from build123d import *

# Parameters (mm, degrees)
SKETCH1_W           = 10.16
SKETCH1_H           = 5.08
SKETCH1_W_2         = 1
SKETCH1_H_2         = 1
BOSS_EXTRUDE2_DEPTH = 8
SKETCH2_W           = 10.16
SKETCH2_H           = 5.08
SKETCH2_R           = 0.5
BOSS_EXTRUDE3_DEPTH = 2
CHAMFER1_SIZE       = 0.2
CHAMFER2_SIZE       = 0.2


with BuildPart() as part:
    # Sketch1 → Boss-Extrude2 (new body)
    with BuildSketch(Plane.XY):
        Rectangle(SKETCH1_W, SKETCH1_H)
        with Locations((-1.27, 1.27)):
            Rectangle(SKETCH1_W_2, SKETCH1_H_2, mode=Mode.SUBTRACT)
        with Locations((-3.81, 1.27)):
            Rectangle(SKETCH1_W_2, SKETCH1_H_2, mode=Mode.SUBTRACT)
        with Locations((1.27, 1.27)):
            Rectangle(SKETCH1_W_2, SKETCH1_H_2, mode=Mode.SUBTRACT)
        with Locations((3.81, 1.27)):
            Rectangle(SKETCH1_W_2, SKETCH1_H_2, mode=Mode.SUBTRACT)
        with Locations((-1.27, -1.27)):
            Rectangle(SKETCH1_W_2, SKETCH1_H_2, mode=Mode.SUBTRACT)
        with Locations((1.27, -1.27)):
            Rectangle(SKETCH1_W_2, SKETCH1_H_2, mode=Mode.SUBTRACT)
        with Locations((3.81, -1.27)):
            Rectangle(SKETCH1_W_2, SKETCH1_H_2, mode=Mode.SUBTRACT)
        with Locations((-3.81, -1.27)):
            Rectangle(SKETCH1_W_2, SKETCH1_H_2, mode=Mode.SUBTRACT)
    extrude(amount=BOSS_EXTRUDE2_DEPTH)

    # Sketch2 → Boss-Extrude3 (add)
    with BuildSketch(Plane.XY.offset(8)):
        Rectangle(SKETCH2_W, SKETCH2_H)
        with Locations((-3.81, 1.27)):
            Circle(SKETCH2_R, mode=Mode.SUBTRACT)
        with Locations((-1.27, 1.27)):
            Circle(SKETCH2_R, mode=Mode.SUBTRACT)
        with Locations((1.27, 1.27)):
            Circle(SKETCH2_R, mode=Mode.SUBTRACT)
        with Locations((3.81, 1.27)):
            Circle(SKETCH2_R, mode=Mode.SUBTRACT)
        with Locations((-1.27, -1.27)):
            Circle(SKETCH2_R, mode=Mode.SUBTRACT)
        with Locations((1.27, -1.27)):
            Circle(SKETCH2_R, mode=Mode.SUBTRACT)
        with Locations((3.81, -1.27)):
            Circle(SKETCH2_R, mode=Mode.SUBTRACT)
        with Locations((-3.81, -1.27)):
            Circle(SKETCH2_R, mode=Mode.SUBTRACT)
    extrude(amount=BOSS_EXTRUDE3_DEPTH)

    # Chamfer1
    chamfer1_edges = [part.edges().sort_by_distance(p)[0] for p in [
        (-4.31, -1.27, 0),
        (-3.81, -1.77, 0),
        (-3.31, -1.27, 0),
        (-3.81, -0.77, 0),
        (-4.31, 1.27, 0),
        (-3.81, 0.77, 0),
        (-3.31, 1.27, 0),
        (-3.81, 1.77, 0),
        (-1.77, 1.27, 0),
        (-1.27, 0.77, 0),
        (-0.77, 1.27, 0),
        (-1.27, 1.77, 0),
        (0.77, 1.27, 0),
        (1.27, 0.77, 0),
        (1.77, 1.27, 0),
        (1.27, 1.77, 0),
        (0, 2.54, 0),
        (5.08, 0, 0),
        (0, -2.54, 0),
        (3.31, 1.27, 0),
        (3.81, 0.77, 0),
        (4.31, 1.27, 0),
        (3.81, 1.77, 0),
        (-5.08, 0, 0),
        (-1.77, -1.27, 0),
        (-1.27, -1.77, 0),
        (-0.77, -1.27, 0),
        (-1.27, -0.77, 0),
        (0.77, -1.27, 0),
        (1.27, -1.77, 0),
        (1.77, -1.27, 0),
        (1.27, -0.77, 0),
        (3.31, -1.27, 0),
        (3.81, -1.77, 0),
        (4.31, -1.27, 0),
        (3.81, -0.77, 0),
    ]]
    chamfer(chamfer1_edges, length=CHAMFER1_SIZE)

    # Chamfer2
    chamfer2_edges = [part.edges().sort_by_distance(p)[0] for p in [
        (-5.08, 0, 10),
        (0, -2.54, 10),
        (5.08, 0, 10),
        (0, 2.54, 10),
    ]]
    chamfer(chamfer2_edges, length=CHAMFER2_SIZE)


solid = part.part
Check sheet for the modelled part. Datum: model origin and axes. Units: mm. A direction names the side the tool comes from. Give positions to 0.01 mm unless a question says otherwise; leave off trailing zeros. Return JSON: item names as keys, results as strings. Group by question number.
1. Thickness scan on L1, parallel to X at y = -1.1, z = 1.75; L2, parallel to Y at x = 3.81, z = 9; L3, parallel to Y at x = -3.5, z = 8.5. Record the ranges inside material, lowest first.
2. Tool access check on faces 3 (the cylindrical face through (-0.808, -1.462, 8.986)), 4 (the flat face through (3.31, -1, 4)). Record the directions out of +Z, -Z, +X, -X, +Y, -Y that give a thin tool (end or side, any length) a straight path to the whole face; none if there is none.
3. Cross-section at A-A on z = 8.5. State how many separate pieces and enclosed holes the cut face has, plus the area to 3 significant figures.
4. Mould release check, pull along X, two halves, no side actions. Record for faces 1 (the flat face through (0, 0, 0)), 2 (the flat face through (-0.77, -1, 4)): released by +X, released by -X, zero draft, split by the parting line, or undercut.
5. Go/stop test with a flat-tipped pin: pin 1 (0.6 mm diameter, centred on x = 1, y = 1, fed in from -Z). Record where the tip stops, or that it passes through.
Return value:
{
 "1": {"L1": "-5.08 to -4.31, -3.31 to -1.77, -0.77 to 0.77, 1.77 to 3.31, 4.31 to 5.08", "L2": "-2.54 to -1.77, -0.77 to 0.77, 1.77 to 2.54", "L3": "-2.54 to -1.66, -0.88 to 0.88, 1.66 to 2.54"},
 "2": {"face 3": "+Z, -Z", "face 4": "-Z"},
 "3": {"separate pieces": "1", "enclosed holes": "8", "area": "45.3 mm^2"},
 "4": {"face 1": "zero draft", "face 2": "undercut"},
 "5": {"pin 1": "z = 0.13"}
}
